```python
from build123d import *

# Parameters (mm, degrees)
SKETCH1_R               = 12.7
BOSS_EXTRUDE1_DEPTH     = 3.175
SKETCH2_R               = 6.35
BOSS_EXTRUDE2_DEPTH     = 1.397
CUT_EXTRUDE1_DEPTH      = 19.533299329
CUT_EXTRUDE1_DEPTH_BACK = 19.533299329
SKETCH3_R               = 1.5
SKETCH4_R               = 1.75
CUT_EXTRUDE2_DEPTH      = 19.238986403
CIRPATTERN1_COUNT       = 8
SKETCH5_R               = 2.5
CUT_EXTRUDE3_DEPTH      = 2.5


with BuildPart() as part:
    # Sketch1 → Boss-Extrude1 (new body)
    with BuildSketch(Plane(origin=(0, 0, 0), x_dir=(1, 0, 0), z_dir=(0, 1, 0))):
        with Locations(Location((0, 0, 0), (0, 0, 270))):
            Circle(SKETCH1_R)
    extrude(amount=-BOSS_EXTRUDE1_DEPTH)

    # Sketch2 → Boss-Extrude2 (add)
    with BuildSketch(Plane(origin=(0, 0, 0), x_dir=(1, 0, 0), z_dir=(0, 1, 0))):
        with Locations(Location((0, 0, 0), (0, 0, 270))):
            Circle(SKETCH2_R)
    extrude(amount=BOSS_EXTRUDE2_DEPTH)

    # Sketch3 → Cut-Extrude1 (cut, two sides: drawn at the far end of the back side and taken through both)
    with BuildSketch(Plane(origin=(0, 1.397, 0), x_dir=(1, 0, 0), z_dir=(0, 1, 0)).offset(-CUT_EXTRUDE1_DEPTH_BACK)):
        with Locations(Location((0, 0, 0), (0, 0, 270))):
            Circle(SKETCH3_R)
    extrude(amount=CUT_EXTRUDE1_DEPTH + CUT_EXTRUDE1_DEPTH_BACK, mode=Mode.SUBTRACT)

    # Sketch4 → Cut-Extrude2 (cut, symmetric)
    with BuildSketch(Plane(origin=(0, 0, 0), x_dir=(1, 0, 0), z_dir=(0, 1, 0))):
        with Locations(Location((0, -9.779, 0), (0, 0, 270))):
            Circle(SKETCH4_R)
    cut_extrude2 = extrude(amount=CUT_EXTRUDE2_DEPTH, both=True, mode=Mode.SUBTRACT)

    # CirPattern1: Cut-Extrude2 ×8 about axis
    cirpattern1_axis = Axis((0, 0, 0), (0, 1, 0))
    for i in range(1, CIRPATTERN1_COUNT):
        add(cut_extrude2.rotate(cirpattern1_axis, i * 360 / CIRPATTERN1_COUNT), mode=Mode.SUBTRACT)

    # Sketch5 → Cut-Extrude3 (cut)
    with BuildSketch(Plane.XZ.offset(3.175)):
        with Locations(Location((0, 0, 0), (0, 0, 270))):
            Circle(SKETCH5_R)
    extrude(amount=-CUT_EXTRUDE3_DEPTH, mode=Mode.SUBTRACT)


solid = part.part
```
Verification items for the finished model (mm, model axes). A direction names the side the tool comes from. Coordinates: 2 decimals unless noted, no trailing zeros. Order: outer loops, then holes, each group sorted by start corner. A loop starts at its lowest first (then second) coordinate and runs counter-clockwise, first axis right, second up. Notation, with made-up numbers: (7, -32.75) - (47, -32.75) arc R24 cw to (47, 1.25) - close; hole circle Ø10 at (39.25, -27). An arc over 180 degrees is marked (long way). Return JSON: item names as keys, results as strings.
(1) Access from +Z, -Z, +X, -X, +Y, -Y to the whole of each face (thin tool, end or side, straight path). Record for faces 4 (the cylindrical face through (-7.7, -1.6, -10.1)), 5 (the cylindrical face through (-2.44, -1.94, 0.54)).
Filled sheet:
{"face 4": "+Y, -Y", "face 5": "-Y"}
(2) Mould release check, pull along X, two halves, no side actions. Record for faces 1 (the flat face through (-3, 0, -6)), 2 (the cylindrical face through (-3.86, 0.69, -5.04)), 3 (the cylindrical face through (5.166, -1.565, -6.839)): pulls with the +X half, pulls with the -X half, needs draft (parallel to the pull), parting line crosses it, or undercut.
Filled sheet:
{"face 1": "needs draft", "face 2": "parting line crosses it", "face 3": "undercut"}
(3) Thickness scan on line 1 along Z through (x, y) = (-1.5, -0.8); line 2 along X through (y, z) = (-0.75, 5.5); line 3 along X through (y, z) = (-1.35, -6.5). Record the ranges inside material, lowest first.
Filled sheet:
{"line 1": "z = -12.61 to -10.68, -8.88 to -2, 2 to 8.88, 10.68 to 12.61", "line 2": "x = -11.45 to -7.94, -5.88 to 5.88, 7.94 to 11.45", "line 3": "x = -10.91 to -8.61, -5.21 to 5.21, 8.61 to 10.91"}
(4) Section check B-B, the plane x = 0. Record the cut outline in (y, z) (3 decimals).
Filled sheet:
{"outline": "(-3.175, -12.7) - (0, -12.7) - (0, -11.529) - (-3.175, -11.529) - close; (-3.175, -8.029) - (0, -8.029) - (0, -6.35) - (1.397, -6.35) - (1.397, -1.5) - (-0.675, -1.5) - (-0.675, -2.5) - (-3.175, -2.5) - close; (-3.175, 2.5) - (-0.675, 2.5) - (-0.675, 1.5) - (1.397, 1.5) - (1.397, 6.35) - (0, 6.35) - (0, 8.029) - (-3.175, 8.029) - close; (-3.175, 11.529) - (0, 11.529) - (0, 12.7) - (-3.175, 12.7) - close"}
(5) Section check C-C, the plane z = -7. Record the cut outline in (x, y) (3 decimals).
Filled sheet:
{"outline": "(-10.597, -3.175) - (-8.663, -3.175) - (-8.663, 0) - (-10.597, 0) - close; (-5.167, -3.175) - (5.167, -3.175) - (5.167, 0) - (-5.167, 0) - close; (8.663, -3.175) - (10.597, -3.175) - (10.597, 0) - (8.663, 0) - close"}
(6) Go/stop test with flat-tipped pins: pin 1 (3 mm diameter, centred on x = 9.779, z = 0, fed in from -Y); pin 2 (4 mm diameter, centred on x = -6.91, z = 6.91, fed in from +Y); pin 3 (1 mm diameter, centred on y = -1.5, z = 8, fed in from -X); pin 4 (4 mm diameter, centred on x = 0, z = 0, fed in from -Y) (3 decimals). Record where each tip stops, or that it passes through.
Filled sheet:
{"pin 1": "passes through", "pin 2": "stops at y = 0", "pin 3": "stops at x = -10.25", "pin 4": "stops at y = -0.675"}
(7) Section check D-D, the plane y = 0.65. Record the cut outline in (x, z).
Filled sheet:
{"outline": "circle Ø12.7 at (0, 0); hole circle Ø3 at (0, 0)"}
(8) Section check A-A, the plane z = 0. Record the cut outline in (x, y) (3 decimals).
Filled sheet:
{"outline": "(-12.7, -3.175) - (-11.529, -3.175) - (-11.529, 0) - (-12.7, 0) - close; (-8.029, -3.175) - (-2.5, -3.175) - (-2.5, -0.675) - (-1.5, -0.675) - (-1.5, 1.397) - (-6.35, 1.397) - (-6.35, 0) - (-8.029, 0) - close; (1.5, -0.675) - (2.5, -0.675) - (2.5, -3.175) - (8.029, -3.175) - (8.029, 0) - (6.35, 0) - (6.35, 1.397) - (1.5, 1.397) - close; (11.529, -3.175) - (12.7, -3.175) - (12.7, 0) - (11.529, 0) - close"}
